Can you work these out from the drawing? Everything is in mm from the part's minimum corner. A direction names the side the tool comes from. Round coordinates to 2 decimals unless told otherwise and drop trailing zeros. Write each loop counter-clockwise with the first axis right and the second up, starting at its lowest first coordinate (ties: lowest second). Pieces come first, ordered by that corner, then holes. Notation, with made-up numbers: (72.25, 14) -> (120.25, 14) arc R20 ccw to (120.25, 46) -> close; hole circle Ø4 at (-10.75, 36.25). An arc over 180 degrees is marked (long way). Write item = value, one per line. Start each with the question number.
1) Imagine slicing it at D-D, the plane z = 24.5. Please give me the cut outline in (x, y), then the cut area to 3 significant figures.
2) Imagine slicing it at B-B, the plane x = 3. Please give me the cut outline in (y, z), then the cut area to 3 significant figures.
3) Imagine slicing it at C-C, the plane y = 2.7. Please give me the cut outline in (x, z), then the cut area to 3 significant figures.
4) I'm going to push a flat-ended pin straight in: pin 1 (2.5 mm diameter, centred on x = 3, z = 4.5, fed in from +Y). Where does the tip first touch, or does it pass through?
5) Imagine slicing it at A-A, the plane z = 4.5. Please give me the cut outline in (x, y), then the cut area to 3 significant figures.
6) Thinking about a two-plate mould opening in Z: for the marked faces 3, 4 and 5, which applies, +Z half, -Z half, draft (parallel to the pull), parting line (faces both ways), or undercut?
7) If I drill on line 1 (Z direction, x = 3, y = 2.2); line 2 (X direction, y = 2.95, z = 36.5); line 3 (X direction, y = 2.1, z = 22), over which ranges is the centre line in solid material (lowest first)?
8) For the marked faces 1 and 2, which set-ups out of +Z, -Z, +X, -X, +Y, -Y let a thin tool reach every point of the face, with its end or its side?
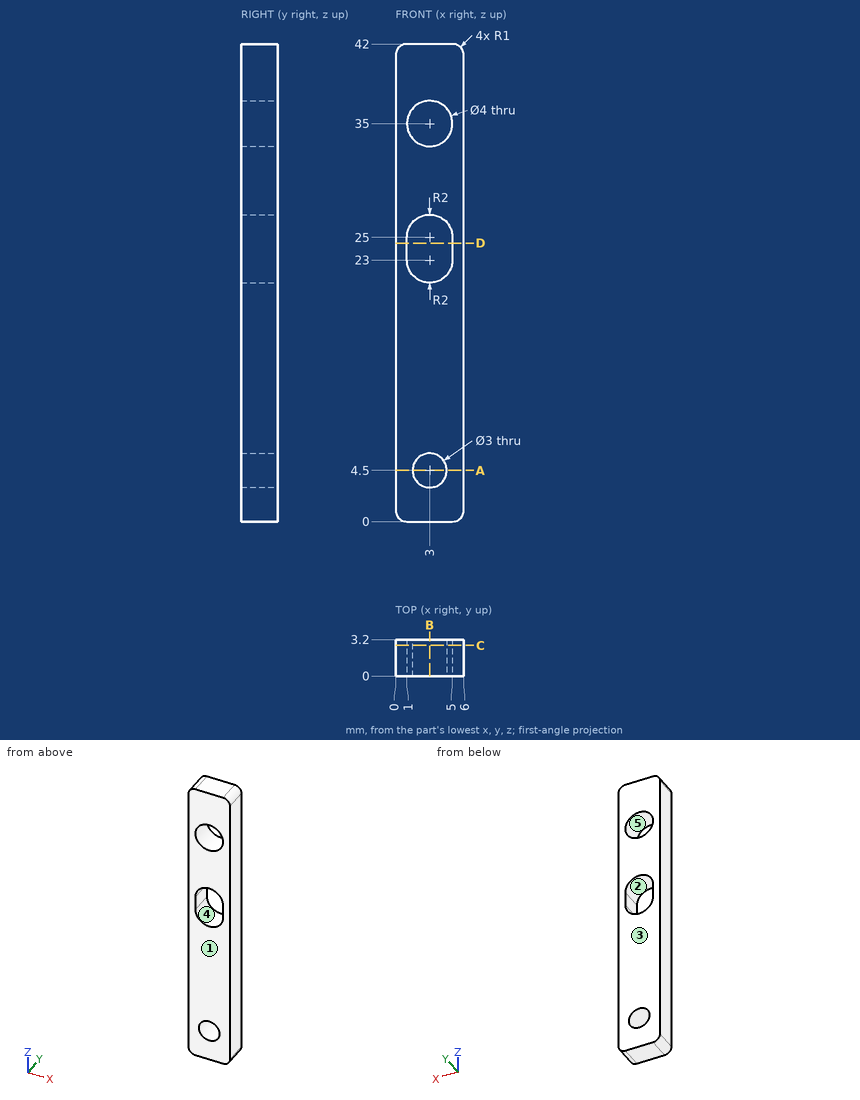
Reported:
q1.outline = (0, 0) -> (1, 0) -> (1, 3.2) -> (0, 3.2) -> close; (5, 0) -> (6, 0) -> (6, 3.2) -> (5, 3.2) -> close
q1.area = 6.40 mm²
q2.outline = (0, 0) -> (3.2, 0) -> (3.2, 3) -> (0, 3) -> close; (0, 6) -> (3.2, 6) -> (3.2, 21) -> (0, 21) -> close; (0, 27) -> (3.2, 27) -> (3.2, 33) -> (0, 33) -> close; (0, 37) -> (3.2, 37) -> (3.2, 42) -> (0, 42) -> close
q2.area = 92.8 mm²
q3.outline = (0, 1) arc R1 ccw to (1, 0) -> (5, 0) arc R1 ccw to (6, 1) -> (6, 41) arc R1 ccw to (5, 42) -> (1, 42) arc R1 ccw to (0, 41) -> close; hole (1, 23) arc R2 ccw to (5, 23) -> (5, 25) arc R2 ccw to (1, 25) -> close; hole circle Ø4 at (3, 35); hole circle Ø3 at (3, 4.5)
q3.area = 211 mm²
q4.pin_1 = through
q5.outline = (0, 0) -> (1.5, 0) -> (1.5, 3.2) -> (0, 3.2) -> close; (4.5, 0) -> (6, 0) -> (6, 3.2) -> (4.5, 3.2) -> close
q5.area = 9.60 mm²
q6.face_3 = draft
q6.face_4 = undercut
q6.face_5 = undercut
q7.line_1 = 0 to 3, 6 to 21, 27 to 33, 37 to 42
q7.line_2 = 0 to 1.68, 4.32 to 6
q7.line_3 = 0 to 1.27, 4.73 to 6
q8.face_1 = +Z, -Z, +X, -X, -Y
q8.face_2 = +Y, -Y
